Build history of the part. All positions in model axes, mm. A direction names the side the tool comes from. Round coordinates to 2 decimals unless told otherwise and drop trailing zeros. Write each loop counter-clockwise with the first axis right and the second up, starting at its lowest first coordinate (ties: lowest second). Pieces come first, ordered by that corner, then holes. Notation, with made-up numbers: (56.5, -19.5) - (67.5, -19.5) arc R19 cw to (67.5, 9.5) - close; hole circle Ø6 at (-10.5, -12.5). An arc over 180 degrees is marked (long way). Answer as a JSON object with one key per item and string values. Group by question number.
Item 1: Slice it at A-A, the plane x = 0. List the corners of the cut face in (y, z) (3 decimals), then the cut area to 3 significant figures.
Item 2: Slice it at B-B, the plane y = -8.5. List the corners of the cut face in (x, z).
Item 3: Which spindle directions (+Z, -Z, +X, -X, +Y, -Y) get a long thin tool onto all of the face, cutting with end or side? Do faces 1 (the cylindrical face through (-5.175, 39.412, 17.395)), 2 (the cylindrical face through (0.202, 52.787, 6.198)), 3 (the flat face through (-16, 39, 2.5)). Say none if no direction does.
Item 4: Probe line 1 (Y direction, x = 0, z = 5.25); line 2 (X direction, y = -1, z = 23.5); line 3 (X direction, y = 16, z = -6). List the from-to ranges inside material, lowest first. Write a range as from..to.
Item 5: Flat gauge pins, fed straight in: pin 1 (4 mm diameter, centred on x = 36.24, y = 36.24, fed in from +Z); pin 2 (1.5 mm diameter, centred on y = -9.5, z = 8, fed in from -X); pin 3 (5 mm diameter, centred on y = -41, z = -1, fed in from -X). Where does each tip first touch, or does it go through?
Item 6: Two-plate mould, pull along Y, no slides. Class faces 4 (the cylindrical face through (-11.923, -53.692, 6.302)), 5 (the flat face through (31, 11, -10)), 6 (the cylindrical face through (16.455, -37.813, -3.838)), 7 (the flat face through (-14, -22, 5)): +Y half, -Y half, draft (parallel to the pull), parting line (faces both ways), or undercut.
Item 7: Slice it at C-C, the plane x = -22. List the corners of the cut face in (y, z).
Item 8: Slice it at D-D, the plane z = 13. List the corners of the cut face in (x, y).
from build123d import *

# Parameters (mm, degrees)
IZIM1_R                     = 55
Y_KSEKLIK_EKSTR_ZYON1_DEPTH = 10
IZIM2_OUTSIDE_W             = 143.368
IZIM2_OUTSIDE_H             = 143.368
IZIM2_OUTSIDE_R             = 47.5
KES_EKSTR_ZYON1_DEPTH       = 12.5
IZIM3_R                     = 1.55
KES_EKSTR_ZYON2_DEPTH       = 79.779756283
DAIRESEL_KAPLAMA1_COUNT     = 8
IZIM5_R                     = 32.525
KES_EKSTR_ZYON3_DEPTH       = 15
IZIM6_R                     = 25.5
KES_EKSTR_ZYON4_DEPTH       = 80.214897589
IZIM7_R                     = 39.75
IZIM7_R_2                   = 25.5
Y_KSEKLIK_EKSTR_ZYON2_DEPTH = 15
IZIM8_R                     = 1.5
IZIM8_R_2                   = 1.464466486
KES_EKSTR_ZYON5_DEPTH       = 12.5


with BuildPart() as part:
    # Çizim1 → Yükseklik-Ekstrüzyon1 (new, symmetric)
    with BuildSketch(Plane.XY):
        Circle(IZIM1_R)
    extrude(amount=Y_KSEKLIK_EKSTR_ZYON1_DEPTH, both=True)

    # Çizim2 outside → Kes-Ekstrüzyon1 (cut)
    with BuildSketch(Plane(origin=(0, 0, -10), x_dir=(-1, 0, 0), z_dir=(0, 0, -1))):
        Rectangle(IZIM2_OUTSIDE_W, IZIM2_OUTSIDE_H)
        Circle(IZIM2_OUTSIDE_R, mode=Mode.SUBTRACT)
    extrude(amount=-KES_EKSTR_ZYON1_DEPTH, mode=Mode.SUBTRACT)

    # Çizim3 → Kes-Ekstrüzyon2 (cut, through all)
    with BuildSketch(Plane(origin=(0, 0, 2.5), x_dir=(-1, 0, 0), z_dir=(0, 0, -1))):
        with Locations((0, 51.25)):
            Circle(IZIM3_R)
    kes_ekstr_zyon2 = extrude(amount=-KES_EKSTR_ZYON2_DEPTH, mode=Mode.SUBTRACT)

    # Dairesel Kaplama1: Kes-Ekstrüzyon2 ×8 about axis
    dairesel_kaplama1_axis = Axis((0, 0, 0), (0, 0, 1))
    for i in range(1, DAIRESEL_KAPLAMA1_COUNT):
        add(kes_ekstr_zyon2.rotate(dairesel_kaplama1_axis, i * 360 / DAIRESEL_KAPLAMA1_COUNT), mode=Mode.SUBTRACT)

    # Çizim5 → Kes-Ekstrüzyon3 (cut)
    with BuildSketch(Plane(origin=(0, 0, -10), x_dir=(-1, 0, 0), z_dir=(0, 0, -1))):
        Circle(IZIM5_R)
    extrude(amount=-KES_EKSTR_ZYON3_DEPTH, mode=Mode.SUBTRACT)

    # Çizim6 → Kes-Ekstrüzyon4 (cut, through all)
    with BuildSketch(Plane(origin=(0, 0, 5), x_dir=(-1, 0, 0), z_dir=(0, 0, -1))):
        Circle(IZIM6_R)
    extrude(amount=-KES_EKSTR_ZYON4_DEPTH, mode=Mode.SUBTRACT)

    # Çizim7 → Yükseklik-Ekstrüzyon2 (add)
    with BuildSketch(Plane.XY.offset(10)):
        Circle(IZIM7_R)
        with Locations(Location((0, 0, 0), (0, 0, 180))):
            Circle(IZIM7_R_2, mode=Mode.SUBTRACT)
    extrude(amount=Y_KSEKLIK_EKSTR_ZYON2_DEPTH)

    # Çizim8 → Kes-Ekstrüzyon5 (cut)
    with BuildSketch(Plane(origin=(0, 0, -10), x_dir=(-1, 0, 0), z_dir=(0, 0, -1))):
        with Locations((16.264045876, -39.264880132)):
            Circle(IZIM8_R)
        with Locations((39.264880132, -16.264045876)):
            Circle(IZIM8_R)
        with Locations((-16.264045876, -39.264880132)):
            Circle(IZIM8_R_2)
        with Locations((-39.264880132, -16.264045876)):
            Circle(IZIM8_R)
        with Locations((39.264880132, 16.264045876)):
            Circle(IZIM8_R)
        with Locations((16.264045876, 39.264880132)):
            Circle(IZIM8_R)
        with Locations((-16.264045876, 39.264880132)):
            Circle(IZIM8_R)
        with Locations((-39.264880132, 16.264045876)):
            Circle(IZIM8_R)
    extrude(amount=-KES_EKSTR_ZYON5_DEPTH, mode=Mode.SUBTRACT)


solid = part.part
Geometry says:
{
 "1": {"outline": "(-55, 2.5) - (-52.8, 2.5) - (-52.8, 10) - (-55, 10) - close; (-49.7, 2.5) - (-47.5, 2.5) - (-47.5, -10) - (-32.525, -10) - (-32.525, 5) - (-25.5, 5) - (-25.5, 25) - (-39.75, 25) - (-39.75, 10) - (-49.7, 10) - close; (25.5, 5) - (32.525, 5) - (32.525, -10) - (47.5, -10) - (47.5, 2.5) - (49.7, 2.5) - (49.7, 10) - (39.75, 10) - (39.75, 25) - (25.5, 25) - close; (52.8, 2.5) - (55, 2.5) - (55, 10) - (52.8, 10) - close", "area": "1,160 mm^2"},
 "2": {"outline": "(-54.34, 2.5) - (-46.73, 2.5) - (-46.73, -10) - (-31.39, -10) - (-31.39, 5) - (-24.04, 5) - (-24.04, 25) - (-38.83, 25) - (-38.83, 10) - (-54.34, 10) - close; (24.04, 5) - (31.39, 5) - (31.39, -10) - (46.73, -10) - (46.73, 2.5) - (54.34, 2.5) - (54.34, 10) - (38.83, 10) - (38.83, 25) - (24.04, 25) - close"},
 "3": {"face 1": "+Z", "face 2": "+Z, -Z", "face 3": "-Z"},
 "4": {"line 1": "y = -55..-52.8, -49.7..-25.5, 25.5..49.7, 52.8..55", "line 2": "x = -39.74..-25.48, 25.48..39.74", "line 3": "x = -44.72..-40.74, -37.79..-28.32, 28.32..37.79, 40.74..44.72"},
 "5": {"pin 1": "stops at z = 10", "pin 2": "stops at x = -54.3", "pin 3": "stops at x = -27.82"},
 "6": {"face 4": "parting line", "face 5": "draft", "face 6": "undercut", "face 7": "undercut"},
 "7": {"outline": "(-50.41, 2.5) - (-42.1, 2.5) - (-42.1, -10) - (-23.96, -10) - (-23.96, 5) - (-12.89, 5) - (-12.89, 25) - (-33.11, 25) - (-33.11, 10) - (-50.41, 10) - close; (12.89, 5) - (23.96, 5) - (23.96, -10) - (42.1, -10) - (42.1, 2.5) - (50.41, 2.5) - (50.41, 10) - (33.11, 10) - (33.11, 25) - (12.89, 25) - close"},
 "8": {"outline": "circle Ø79.5 at (0, 0); hole circle Ø51 at (0, 0)"}
}
